```python
from build123d import *

# Parameters (mm, degrees)
SKETCH2_W           = 112.00010125
SKETCH2_H           = 190.5995575
SKETCH2_R           = 2.1
SKETCH2_R_2         = 1.85
BOSS_EXTRUDE1_DEPTH = 1.2
SKETCH5_W           = 2
SKETCH5_H           = 37.6
SKETCH5_H_2         = 0.6
CUT_EXTRUDE2_DEPTH  = 247.246128205
CUT_EXTRUDE1_DEPTH  = 247.246128205
SKETCH9_W           = 14
SKETCH9_H           = 3.4
SKETCH9_W_2         = 8.5
BOSS_EXTRUDE5_DEPTH = 1.2
FILLET1_R           = 1
CUT_EXTRUDE4_REACH  = 248.246
SKETCH10_W          = 8.2
SKETCH10_H          = 0.7
SKETCH11_R          = 2.25
CUT_EXTRUDE5_DEPTH  = 247.246128205
BOSS_EXTRUDE6_DEPTH = 1.2
SKETCH13_R          = 1.635773904
CUT_EXTRUDE6_DEPTH  = 248.202612706
SKETCH15_W          = 166.29246115
SKETCH15_H          = 51.52086731
CUT_EXTRUDE7_DEPTH  = 10
SKETCH17_R          = 1.65
BOSS_EXTRUDE7_DEPTH = 1.2
BOSS_EXTRUDE8_START = -1.2
SKETCH18_R          = 1.65
BOSS_EXTRUDE8_DEPTH = 1.2
BOSS_EXTRUDE9_START = -1.2
SKETCH19_R          = 4
BOSS_EXTRUDE9_DEPTH = 1.2
FILLET3_R           = 5
FILLET8_R           = 10
FILLET10_R          = 5


with BuildPart() as part:
    # Sketch2 → Boss-Extrude1 (new body)
    with BuildSketch(Plane.XY):
        with Locations((50.167238625, 126.88082875)):
            Rectangle(SKETCH2_W, SKETCH2_H)
        with Locations((8.16763175, 151.180160625)):
            Circle(SKETCH2_R, mode=Mode.SUBTRACT)
        with Locations((100.1668405, 151.180160625)):
            Circle(SKETCH2_R_2, mode=Mode.SUBTRACT)
        with Locations((100.1668405, 36.181495)):
            Circle(SKETCH2_R_2, mode=Mode.SUBTRACT)
        with Locations((8.16763175, 36.181495)):
            Circle(SKETCH2_R, mode=Mode.SUBTRACT)
    extrude(amount=BOSS_EXTRUDE1_DEPTH)

    # Sketch5 → Cut-Extrude2 (cut, through all)
    with BuildSketch(Plane.XY.offset(1.2)):
        Polygon((-3.832812, 185.1806075), (6.667188, 185.1806075), (6.667188, 222.1806075), (-5.832812, 222.1806075), (-5.832812, 185.1806075), (-5.832812, 184.5806075), (-3.832812, 184.5806075), align=None)
        with Locations((105.16728925, 203.3806075)):
            Rectangle(SKETCH5_W, SKETCH5_H)
        with Locations((-4.832812, 31.88105)):
            Rectangle(SKETCH5_W, SKETCH5_H_2)
        with Locations((105.16728925, 31.88105)):
            Rectangle(SKETCH5_W, SKETCH5_H_2)
    extrude(amount=-CUT_EXTRUDE2_DEPTH, mode=Mode.SUBTRACT)

    # Sketch4 → Cut-Extrude1 (cut, through all)
    with BuildSketch(Plane.XY.offset(1.2)):
        with BuildLine():
            Line((55.16728925, 218.1806075), (98.16728925, 218.1806075))
            ThreePointArc((98.16728925, 218.1806075), (99.581502812, 217.594821062), (100.16728925, 216.1806075))
            Line((100.16728925, 216.1806075), (100.16728925, 192.1806075))
            ThreePointArc((100.16728925, 192.1806075), (99.581502812, 190.766393938), (98.16728925, 190.1806075))
            Line((98.16728925, 190.1806075), (55.16728925, 190.1806075))
            ThreePointArc((55.16728925, 190.1806075), (53.753075688, 190.766393938), (53.16728925, 192.1806075))
            Line((53.16728925, 192.1806075), (53.16728925, 216.1806075))
            ThreePointArc((53.16728925, 216.1806075), (53.753075688, 217.594821062), (55.16728925, 218.1806075))
        make_face()
    extrude(amount=-CUT_EXTRUDE1_DEPTH, mode=Mode.SUBTRACT)

    # Sketch9 → Boss-Extrude5 (add)
    with BuildSketch(Plane.XY.offset(1.2)):
        with Locations((5.167188, 29.88105)):
            Rectangle(SKETCH9_W, SKETCH9_H)
        with Locations((95.16728925, 29.88105)):
            Rectangle(SKETCH9_W, SKETCH9_H)
        with Locations((50.167238625, 29.88105)):
            Rectangle(SKETCH9_W, SKETCH9_H)
        with Locations((2.417188, 186.8806075)):
            Rectangle(SKETCH9_W_2, SKETCH9_H)
    extrude(amount=-BOSS_EXTRUDE5_DEPTH)

    # Fillet1
    fillet1_edges = [part.edges().sort_by_distance(p)[0] for p in [
        (102.16728925, 28.18105, 0.6),
        (88.16728925, 28.18105, 0.6),
        (57.167238625, 28.18105, 0.6),
        (43.167238625, 28.18105, 0.6),
        (12.167188, 28.18105, 0.6),
        (-1.832812, 28.18105, 0.6),
        (-1.832812, 188.5806075, 0.6),
    ]]
    fillet(fillet1_edges, radius=FILLET1_R)

    # Sketch10 → Cut-Extrude4 (cut, up to next)
    with BuildSketch(Plane.XY.offset(1.2), mode=Mode.PRIVATE) as cut_extrude4_sk1:
        with Locations((95.16728925, 31.93105)):
            Rectangle(SKETCH10_W, SKETCH10_H)
    cut_extrude4_tool1 = extrude(cut_extrude4_sk1.sketch, amount=-CUT_EXTRUDE4_REACH, mode=Mode.PRIVATE) & part.part
    # Sketch10 → Cut-Extrude4 (cut, up to next)
    with BuildSketch(Plane.XY.offset(1.2), mode=Mode.PRIVATE) as cut_extrude4_sk2:
        with Locations((50.167238625, 31.93105)):
            Rectangle(SKETCH10_W, SKETCH10_H)
    cut_extrude4_tool2 = extrude(cut_extrude4_sk2.sketch, amount=-CUT_EXTRUDE4_REACH, mode=Mode.PRIVATE) & part.part
    # Sketch10 → Cut-Extrude4 (cut, up to next)
    with BuildSketch(Plane.XY.offset(1.2), mode=Mode.PRIVATE) as cut_extrude4_sk3:
        with Locations((5.167188, 31.93105)):
            Rectangle(SKETCH10_W, SKETCH10_H)
    cut_extrude4_tool3 = extrude(cut_extrude4_sk3.sketch, amount=-CUT_EXTRUDE4_REACH, mode=Mode.PRIVATE) & part.part
    # Sketch10 → Cut-Extrude4 (cut, up to next)
    with BuildSketch(Plane.XY.offset(1.2), mode=Mode.PRIVATE) as cut_extrude4_sk4:
        with Locations((50.167238625, 184.8306075)):
            Rectangle(SKETCH10_W, SKETCH10_H)
    cut_extrude4_tool4 = extrude(cut_extrude4_sk4.sketch, amount=-CUT_EXTRUDE4_REACH, mode=Mode.PRIVATE) & part.part
    # Sketch10 → Cut-Extrude4 (cut, up to next)
    with BuildSketch(Plane.XY.offset(1.2), mode=Mode.PRIVATE) as cut_extrude4_sk5:
        with Locations((95.16728925, 184.8306075)):
            Rectangle(SKETCH10_W, SKETCH10_H)
    cut_extrude4_tool5 = extrude(cut_extrude4_sk5.sketch, amount=-CUT_EXTRUDE4_REACH, mode=Mode.PRIVATE) & part.part
    # Sketch10 → Cut-Extrude4 (cut, up to next)
    with BuildSketch(Plane.XY.offset(1.2), mode=Mode.PRIVATE) as cut_extrude4_sk6:
        with Locations((5.167188, 184.8306075)):
            Rectangle(SKETCH10_W, SKETCH10_H)
    cut_extrude4_tool6 = extrude(cut_extrude4_sk6.sketch, amount=-CUT_EXTRUDE4_REACH, mode=Mode.PRIVATE) & part.part
    add(cut_extrude4_tool1.solids().sort_by_distance((95.167289, 31.93105, 1.2))[0], mode=Mode.SUBTRACT)
    add(cut_extrude4_tool2.solids().sort_by_distance((50.167239, 31.93105, 1.2))[0], mode=Mode.SUBTRACT)
    add(cut_extrude4_tool3.solids().sort_by_distance((5.167188, 31.93105, 1.2))[0], mode=Mode.SUBTRACT)
    add(cut_extrude4_tool4.solids().sort_by_distance((50.167239, 184.830607, 1.2))[0], mode=Mode.SUBTRACT)
    add(cut_extrude4_tool5.solids().sort_by_distance((95.167289, 184.830607, 1.2))[0], mode=Mode.SUBTRACT)
    add(cut_extrude4_tool6.solids().sort_by_distance((5.167188, 184.830607, 1.2))[0], mode=Mode.SUBTRACT)

    # Sketch11 → Cut-Extrude5 (cut, through all)
    with BuildSketch(Plane.XY.offset(1.2)):
        with Locations((61.367697375, 160.67994375)):
            Circle(SKETCH11_R)
        with Locations((13.067697375, 172.47994375)):
            Circle(SKETCH11_R)
        with BuildLine():
            Line((71.867697375, 175.27994375), (71.867697375, 170.27994375))
            ThreePointArc((71.867697375, 170.27994375), (69.367697375, 167.77994375), (66.867697375, 170.27994375))
            Line((66.867697375, 170.27994375), (66.867697375, 175.27994375))
            ThreePointArc((66.867697375, 175.27994375), (69.367697375, 177.77994375), (71.867697375, 175.27994375))
        make_face()
    extrude(amount=-CUT_EXTRUDE5_DEPTH, mode=Mode.SUBTRACT)

    # Sketch12 → Boss-Extrude6 (add)
    with BuildSketch(Plane.XY.offset(1.2)):
        with BuildLine():
            Line((104.16728925, 222.1806075), (104.16728925, 213.7806075))
            ThreePointArc((104.16728925, 213.7806075), (108.36728925, 217.9806075), (104.16728925, 222.1806075))
        make_face()
    extrude(amount=-BOSS_EXTRUDE6_DEPTH)

    # Sketch13 → Cut-Extrude6 (cut, through all)
    with BuildSketch(Plane.XY.offset(1.2)):
        with Locations((104.16728925, 217.9806075)):
            Circle(SKETCH13_R)
        with Locations((47.16728925, 217.9806075)):
            Circle(SKETCH13_R)
        with Locations((10.667188, 217.9806075)):
            Circle(SKETCH13_R)
    extrude(amount=-CUT_EXTRUDE6_DEPTH, mode=Mode.SUBTRACT)

    # Sketch15 → Cut-Extrude7 (cut)
    with BuildSketch(Plane.XY.offset(1.2)):
        with Locations((89.813418575, 214.341041155)):
            Rectangle(SKETCH15_W, SKETCH15_H)
    extrude(amount=-CUT_EXTRUDE7_DEPTH, mode=Mode.SUBTRACT)

    # Sketch17 → Boss-Extrude7 (add)
    # profile 1 of 2: a face of its own
    with BuildSketch(Plane(origin=(0, 0, 0), x_dir=(-1, 0, 0), z_dir=(0, 0, -1))):
        with BuildLine():
            Line((-81.1668405, 188.5806075), (-95.1668405, 188.5806075))
            ThreePointArc((-95.1668405, 188.5806075), (-92.691966766, 189.605733766), (-91.6668405, 192.0806075))
            Line((-91.6668405, 192.0806075), (-91.6668405, 194.093254991))
            ThreePointArc((-91.6668405, 194.093254991), (-88.1668405, 197.593254991), (-84.6668405, 194.093254991))
            Line((-84.6668405, 194.093254991), (-84.6668405, 192.0806075))
            ThreePointArc((-84.6668405, 192.0806075), (-83.641714234, 189.605733766), (-81.1668405, 188.5806075))
        make_face()
        with Locations((-88.1668405, 194.093254991)):
            Circle(SKETCH17_R, mode=Mode.SUBTRACT)
    # profile 2 of 2: a face of its own
    with BuildSketch(Plane(origin=(0, 0, 0), x_dir=(-1, 0, 0), z_dir=(0, 0, -1))):
        with BuildLine():
            Line((-19.6668405, 188.5806075), (-33.6668405, 188.5806075))
            ThreePointArc((-33.6668405, 188.5806075), (-31.191966766, 189.605733766), (-30.1668405, 192.0806075))
            Line((-30.1668405, 192.0806075), (-30.1668405, 194.093254991))
            ThreePointArc((-30.1668405, 194.093254991), (-26.6668405, 197.593254991), (-23.1668405, 194.093254991))
            Line((-23.1668405, 194.093254991), (-23.1668405, 192.0806075))
            ThreePointArc((-23.1668405, 192.0806075), (-22.141714234, 189.605733766), (-19.6668405, 188.5806075))
        make_face()
        with Locations((-26.6668405, 194.093254991)):
            Circle(SKETCH17_R, mode=Mode.SUBTRACT)
    extrude(amount=-BOSS_EXTRUDE7_DEPTH)

    # Sketch18 → Boss-Extrude8 (add)
    with BuildSketch(Plane.XY.offset(1.2).offset(BOSS_EXTRUDE8_START)):
        with BuildLine():
            Line((89.16728925, 28.18105), (101.16728925, 28.18105))
            ThreePointArc((101.16728925, 28.18105), (101.874396031, 28.473943219), (102.16728925, 29.18105))
            ThreePointArc((102.16728925, 29.18105), (94.810709764, 12.373227692), (77.471885747, 6.374283268))
            ThreePointArc((77.471885747, 6.374283268), (74.292882483, 9.419749119), (76.639173718, 13.144778172))
            ThreePointArc((76.639173718, 13.144778172), (84.986182742, 19.306088457), (88.16728925, 29.18105))
            ThreePointArc((88.16728925, 29.18105), (88.460182469, 28.473943219), (89.16728925, 28.18105))
        make_face()
        with Locations((77.748285655, 9.844733678)):
            Circle(SKETCH18_R, mode=Mode.SUBTRACT)
    extrude(amount=BOSS_EXTRUDE8_DEPTH)

    # Sketch19 → Boss-Extrude9 (add)
    with BuildSketch(Plane.XY.offset(1.2).offset(BOSS_EXTRUDE9_START)):
        with BuildLine():
            Line((63.367697375, 188.5806075), (81.1668405, 188.5806075))
            ThreePointArc((81.1668405, 188.5806075), (83.641714234, 189.605733766), (84.6668405, 192.0806075))
            Line((84.6668405, 192.0806075), (84.6668405, 194.093254991))
            ThreePointArc((84.6668405, 194.093254991), (86.152024438, 196.955162788), (89.347135493, 197.388236588))
            Line((89.347135493, 197.388236588), (71.39106022, 203.820280323))
            ThreePointArc((71.39106022, 203.820280323), (65.913726984, 203.077868093), (63.367697375, 198.171740441))
            Line((63.367697375, 198.171740441), (63.367697375, 188.5806075))
        make_face()
        with Locations((69.367697375, 198.171740441)):
            Circle(SKETCH19_R, mode=Mode.SUBTRACT)
    extrude(amount=BOSS_EXTRUDE9_DEPTH)

    # Fillet3
    fillet3_edges = [part.edges().sort_by_distance(p)[0] for p in [
        (63.367697375, 188.5806075, 0.6),
    ]]
    fillet(fillet3_edges, radius=FILLET3_R)

    # Fillet8
    # the kernel refuses this fillet: 10 mm, written as the material it adds along each edge
    with BuildSketch(Plane(origin=(88.16728925, 31.58105, 1.2), x_dir=(0, -1, 0), z_dir=(0, 0, -1))) as fillet8_piece_1:
        with BuildLine():
            CenterArc((10, 6.499230724), FILLET8_R, 180, 40.535802111)
            Line((0, 6.499230724), (-0.2, 6.499230724))
            Line((-0.2, 6.499230724), (-0.2, 0))
            Line((-0.2, 0), (0, -0.2))
            ThreePointArc((0, -0.2), (1.2, -0.2), (2.248, -0.129984614))
            Line((2.248, -0.129984614), (2.4, 0))
        make_face()
    extrude(amount=1.2)

    # Fillet10
    fillet10_edges = [part.edges().sort_by_distance(p)[0] for p in [
        (88.16728925, 29.18105, 0.6),
    ]]
    fillet(fillet10_edges, radius=FILLET10_R)


solid = part.part
```
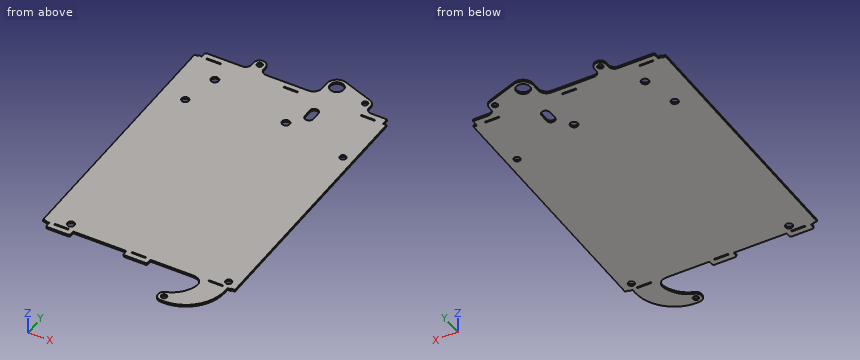
Verification items for the finished model (mm, model axes). Coordinates: 2 decimals unless noted, no trailing zeros. Write each loop counter-clockwise with the first axis right and the second up, starting at its lowest first coordinate (ties: lowest second). Pieces come first, ordered by that corner, then holes. Notation, with made-up numbers: M 37.5,7.5 L 73.5,7.5 A25 cw 73.5,22.5 Z; hole C 55.5,39.25 d10. An arc over 180 degrees is marked long. Answer as a JSON object with one key per item and string values. Group by question number.
(1) Material ranges on line 1 (X direction, y = 195.5, z = 1.1); line 2 (Y direction, x = 77.5, z = 0.5); line 3 (Y direction, x = 96.5, z = 0.9), recorded low to high.
(2) Cross-section at B-B, the plane z = 0.85. State how many separate pieces and enclosed holes the cut face has, and give its area (3 significant figures).
(3) Cross-section at C-C, the plane y = 22. Record the cut outline in (x, z).
(4) Gauge pin test, flat ends, axial feed: pin 1 (0.6 mm diameter, centred on x = -4.5, z = 0.5, fed in from -Y); pin 2 (0.6 mm diameter, centred on x = 71.5, z = 0.5, fed in from -Y); pin 3 (0.6 mm diameter, centred on x = 97, z = 1, fed in from -Y). Record the tip position at first contact, or that the pin passes through.
(5) Cross-section at A-A, the plane x = 36.5. Record the cut outline in (y, z), and give its area (3 significant figures).
Reply:
{
 "1": {"line 1": "23.46 to 25.8, 27.53 to 29.87, 63.37 to 66.39, 72.34 to 87.3, 89.03 to 91.37", "line 2": "6.37 to 8.21, 11.48 to 13.46, 31.58 to 201.63", "line 3": "14.11 to 31.58, 32.28 to 184.48, 185.18 to 188.58"},
 "2": {"separate pieces": "1", "enclosed holes": "17", "area": "18,200 mm²"},
 "3": {"outline": "M 86.57,0 L 101.01,0 L 101.01,1.2 L 86.57,1.2 Z"},
 "4": {"pin 1": "y = 32.18", "pin 2": "y = 31.58", "pin 3": "y = 14.34"},
 "5": {"outline": "M 31.58,0 L 188.58,0 L 188.58,1.2 L 31.58,1.2 Z", "area": "188 mm²"}
}
